Source: CAD feature listing. Evaluate the final solid. Frame: model axes, mm. Face numbers are marked on the shaded views. Round coordinates to 2 decimals unless told otherwise and drop trailing zeros. Loops run counter-clockwise (first coordinate to the right, second up) from the corner with the lowest first, then second, coordinate; pieces in that order, holes last.
Item 1: Ray query, L1, parallel to Z at x = 1, y = 0; L2, parallel to Y at x = 16, z = -20; L3, parallel to Y at x = -13, z = -37.5. Return the intervals inside material, ascending.
Item 2: First-contact query: P1, Ø1, axis at x = -8, z = -43, coming from the -Y side; P2, Ø8, axis at x = -6.5, z = 23, coming from the +Y side; P3, Ø8, axis at x = 11, z = -50, coming from the +Y side. Flat tips, straight axial feed; report the tip coordinate or a pass-through.
Item 3: Pull-direction query (Y, two-part tool) for the marked faces 1, 2 and 3; classes: released by +Y, released by -Y, zero draft, split by the parting line, or undercut.
Item 4: Section query B-B on x = 1.5. Return loops of the section in (y, z).
```python
from build123d import *

# Parameters (mm, degrees)
F2_R    = 5.08
F3_SIZE = 5.08
F4_R    = 5.08


with BuildPart() as f1:
    # F0 (on Front) → F1 (revolve)
    with BuildSketch(Plane.XZ):
        Polygon((19.406605757, 62.1960816438), (-17.702616065, 62.1960816438), (-17.702616065, 43.1460816438), (-4.7324024234, 43.1460816438), (-4.7324024234, -6.6680153832), (-17.702616065, -6.6680153832), (-17.702616065, -14.0039183562), (-4.7324024234, -14.0039183562), (6.4363921154, -14.0039183562), (6.4363921154, 43.1460816438), (19.406605757, 43.1460816438), align=None)
    revolve(axis=Axis((6.8320201244, 0, -20.3539183562), (1, 0, 0)))

    # F2
    f2_edges = [f1.edges().sort_by_distance(p)[0] for p in [
        (-4.732402, 0, -83.853918),
        (6.436392, 0, -83.853918),
        (19.406606, 0, -102.903918),
        (-17.702616, 0, -102.903918),
    ]]
    fillet(f2_edges, radius=F2_R)

    # F3
    f3_edges = [f1.edges().sort_by_distance(p)[0] for p in [
        (19.406606, 0, -83.853918),
    ]]
    chamfer(f3_edges, length=F3_SIZE)

    # F4
    f4_edges = [f1.edges().sort_by_distance(p)[0] for p in [
        (-4.732402, 0, -34.039821),
    ]]
    fillet(f4_edges, radius=F4_R)


solid = f1.part
```
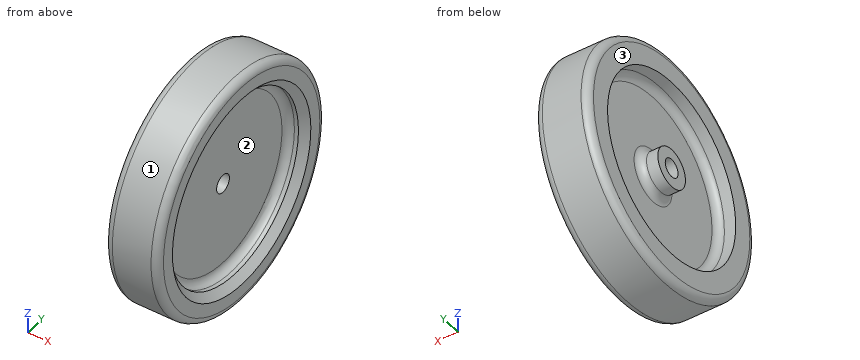
Data:
1. L1: z = -102.9 to -26.7, -14 to 62.2
1. L2: y = -82.27 to -65.17, 65.17 to 82.27
1. L3: y = -80.74 to -61.14, 61.14 to 80.74
2. P1: stops at y = -79.52
2. P2: stops at y = 72.57
2. P3: stops at y = 78.47
3. face 1: split by the parting line
3. face 2: undercut
3. face 3: zero draft
4. outline: circle Ø165.1 at (0, -20.35); hole circle Ø12.7 at (0, -20.35)
